For this review, take the finished solid that the model builds, in its own axes (mm). Face numbers are marked on the shaded views. Round coordinates to 2 decimals unless told otherwise and drop trailing zeros. Write each loop counter-clockwise with the first axis right and the second up, starting at its lowest first coordinate (ties: lowest second). Pieces come first, ordered by that corner, then holes. Notation, with made-up numbers: (65.5, 58) - (111.5, 58) arc R31 ccw to (111.5, 95) - close; hole circle Ø3 at (81, 32). An arc over 180 degrees is marked (long way). Answer in a Markdown table with one row per item. Add a question column.
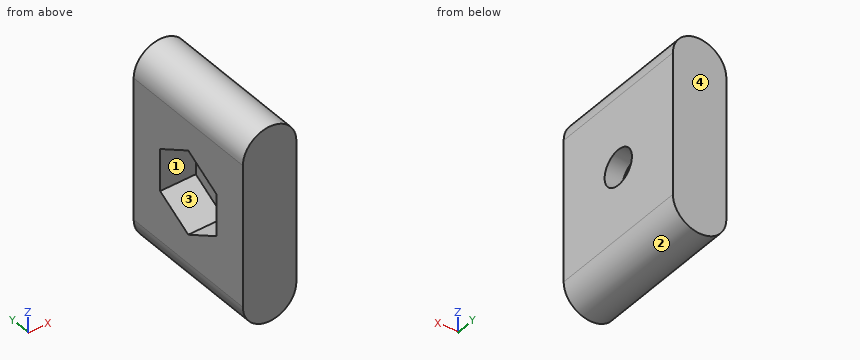
from build123d import *

# Parameters (mm, degrees)
BOSS_EXTRUDE1_DEPTH = 20
SKETCH2_R           = 2.5
CUT_EXTRUDE1_DEPTH  = 20
SKETCH2_4_R         = 2.5
CUT_EXTRUDE2_DEPTH  = 5


with BuildPart() as part:
    # Sketch1 → Boss-Extrude1 (new body)
    with BuildSketch(Plane(origin=(0, 0, 0), x_dir=(1, 0, 0), z_dir=(0, 1, 0))):
        with BuildLine():
            Line((-3.75, -8.45729612), (-3.75, 11.54270388))
            ThreePointArc((-3.75, 11.54270388), (0, 15.29270388), (3.75, 11.54270388))
            Line((3.75, 11.54270388), (3.75, -8.45729612))
            ThreePointArc((3.75, -8.45729612), (0, -12.20729612), (-3.75, -8.45729612))
        make_face()
    extrude(amount=BOSS_EXTRUDE1_DEPTH)

    # Sketch2 → Cut-Extrude1 (cut)
    with BuildSketch(Plane.ZY.offset(3.75)):
        with Locations((-1.54270388, 10)):
            Circle(SKETCH2_R)
    extrude(amount=-CUT_EXTRUDE1_DEPTH, mode=Mode.SUBTRACT)

    # Sketch2<4> → Cut-Extrude2 (cut)
    with BuildSketch(Plane.ZY.offset(3.75)):
        Polygon((4.402095487, 10), (1.429695804, 15.148347272), (-4.515103563, 15.148347272), (-7.487503247, 10), (-4.515103563, 4.851652728), (1.429695804, 4.851652728), align=None)
        with Locations((-1.54270388, 10)):
            Circle(SKETCH2_4_R, mode=Mode.SUBTRACT)
    extrude(amount=-CUT_EXTRUDE2_DEPTH, mode=Mode.SUBTRACT)


solid = part.part
Q1. To check wall thickness, follow probe 1 along Z at (x, y) = (-1, 15); probe 2 along Y at (x, z) = (-0.25, -5); probe 3 along Z at (x, y) = (2, 8). State the ranges of each line that lie inside material, in increasing order.
Q2. Add section D-D on x = 2.5. State the section outline as (y, z) points, then the cut area to 3 significant figures.
Q3. Insertion check: pin 1 Ø6.5 at (y, z) = (10, -1.54) entering from +X; pin 2 Ø2 at (x, y) = (1.5, 8.5) entering from +Z. Each pin has a flat end and moves straight along its axis. Give the tip position at first contact, or say it passes through.
Q4. Add section B-B on y = 13.75. State the section outline as (x, z) points, then the cut area to 3 significant figures.
Q5. Draft analysis for pull direction Z (two halves, no side actions). For the marked faces 1, 2, 3 and 4, state which applies: released by +Z, released by -Z, zero draft, split by the parting line, or undercut.
Q6. Add section A-A on x = 0. State the section outline as (y, z) points, then the cut area to 3 significant figures.
Q7. Add section C-C on z = 3. State the section outline as (x, y) points.
Answer sheet:
| question | item | result |
|---|---|---|
| 1 | probe 1 | z = -15.16 to -4.6, 1.52 to 12.07 |
| 1 | probe 2 | y = 0 to 5.69, 14.31 to 20 |
| 1 | probe 3 | z = -14.71 to -3.04, -0.04 to 11.63 |
| 2 | outline | (0, -14.34) - (20, -14.34) - (20, 11.25) - (0, 11.25) - close; hole circle Ø5 at (10, -1.54) |
| 2 | area | 492 mm² |
| 3 | pin 1 | stops at x = 3.75 |
| 3 | pin 2 | stops at z = 12.17 |
| 4 | outline | (-3.75, -11.54) arc R3.75 ccw to (3.75, -11.54) - (3.75, 8.46) arc R3.75 ccw to (-3.75, 8.46) - (-3.75, 2.24) - (1.25, 2.24) - (1.25, -5.32) - (-3.75, -5.32) - close |
| 4 | area | 156 mm² |
| 5 | face 1 | undercut |
| 5 | face 2 | released by -Z |
| 5 | face 3 | undercut |
| 5 | face 4 | zero draft |
| 6 | outline | (0, -15.29) - (20, -15.29) - (20, 12.21) - (0, 12.21) - close; hole (4.85, -4.52) - (10, -7.49) - (15.15, -4.52) - (15.15, 1.43) - (10, 4.4) - (4.85, 1.43) - close |
| 6 | area | 458 mm² |
| 7 | outline | (-3.75, 0) - (3.75, 0) - (3.75, 20) - (-3.75, 20) - (-3.75, 12.43) - (1.25, 12.43) - (1.25, 7.57) - (-3.75, 7.57) - close |
